Here's the drawing with two shaded views (mm, measured from the low corner). I have some questions. A direction names the side the tool comes from. Give positions to 0.01 mm unless a question says otherwise; leave off trailing zeros. Loops run counter-clockwise (first coordinate to the right, second up) from the corner with the lowest first, then second, coordinate; pieces in that order, holes last. Notation, with made-up numbers: (42, 26) - (90, 26) arc R25 cw to (90, 57) - close; hole circle Ø9 at (-32, 19). An arc over 180 degrees is marked (long way). Use one line per item in the form item = value.
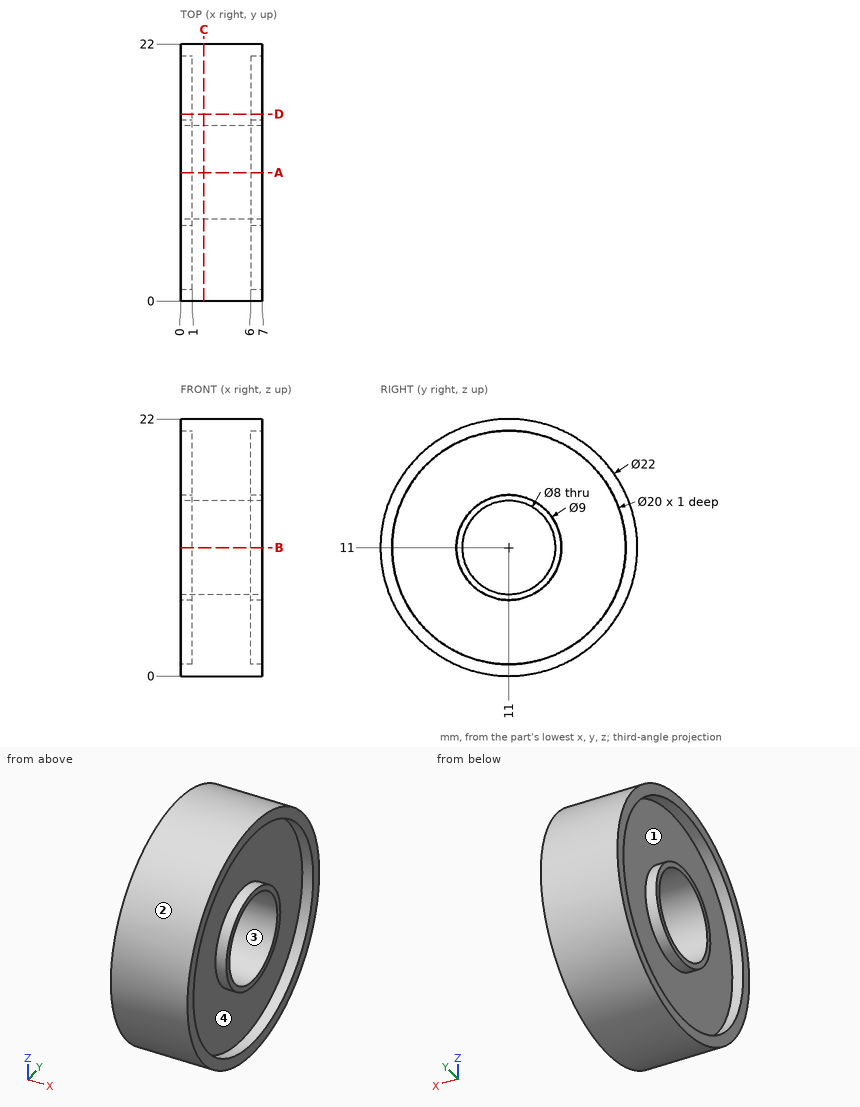
(1) If I drill on probe 1 along Y at (x, z) = (6.45, 11); probe 2 along Y at (x, z) = (4, 11); probe 3 along X at (y, z) = (16.75, 5), over which ranges is the centre line in solid material (lowest first)?
Geometry says:
probe_1 = 0 to 1, 6.5 to 7, 15 to 15.5, 21 to 22
probe_2 = 0 to 7, 15 to 22
probe_3 = 1 to 6
(2) If we section it at C-C (x = 2): List the corners of the cut face in (y, z) for me, plus the area to 3 significant figures.
Geometry says:
outline = circle Ø22 at (11, 11); hole circle Ø8 at (11, 11)
area = 330 mm²
(3) If we section it at A-A (y = 11): List the corners of the cut face in (x, z) for me.
Geometry says:
outline = (0, 0) - (7, 0) - (7, 1) - (6, 1) - (6, 6.5) - (7, 6.5) - (7, 7) - (0, 7) - (0, 6.5) - (1, 6.5) - (1, 1) - (0, 1) - close; (0, 15) - (7, 15) - (7, 15.5) - (6, 15.5) - (6, 21) - (7, 21) - (7, 22) - (0, 22) - (0, 21) - (1, 21) - (1, 15.5) - (0, 15.5) - close
(4) Thinking about a two-plate mould opening in Z: for the marked faces 1 and 2, which applies, pulls with the +Z half, pulls with the -Z half, needs draft (parallel to the pull), parting line crosses it, or undercut?
Geometry says:
face_1 = undercut
face_2 = parting line crosses it
(5) For P1, Ø3, axis at y = 12, z = 14, coming from the +X side; P2, Ø1.5, axis at x = 5, y = 4.5, coming from the +Z side; P3, Ø3, axis at x = 4, z = 19, coming from the +Y side; P4, Ø4, axis at x = 3, y = 4.5, coming from the +Z side, each with a flat end and sliding along its axis, tell me the tip position at first contact or that it passes through.
Geometry says:
P1 = 7
P2 = 20.38
P3 = 19.87
P4 = 21.04
(6) For the marked faces 3 and 4, which set-ups out of +Z, -Z, +X, -X, +Y, -Y let a thin tool reach every point of the face, with its end or its side?
Geometry says:
face_3 = +X, -X
face_4 = +X
(7) If we section it at D-D (y = 16): List the corners of the cut face in (x, z) for me, plus the area to 3 significant figures.
Geometry says:
outline = (0, 1.2) - (7, 1.2) - (7, 2.34) - (6, 2.34) - (6, 19.66) - (7, 19.66) - (7, 20.8) - (0, 20.8) - (0, 19.66) - (1, 19.66) - (1, 2.34) - (0, 2.34) - close
area = 103 mm²
